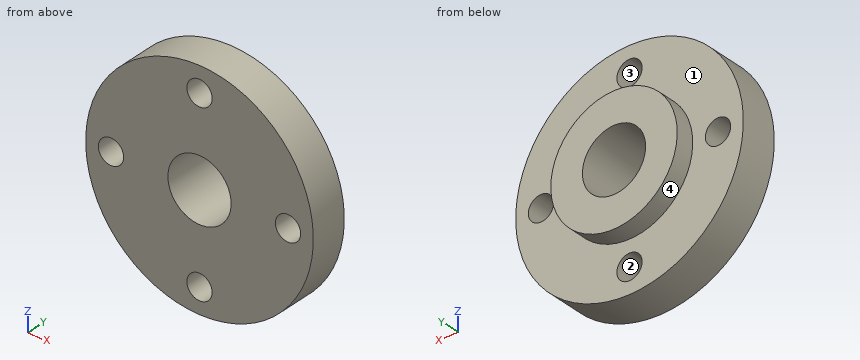
from build123d import *

# Parameters (mm, degrees)
SKETCH1_R           = 36
SKETCH1_R_2         = 10
BOSS_EXTRUDE1_DEPTH = 12
SKETCH2_R           = 20
SKETCH2_R_2         = 10
BOSS_EXTRUDE2_DEPTH = 6
CUT_EXTRUDE1_REACH  = 54.307
SKETCH3_R           = 4


with BuildPart() as part:
    # Sketch1 → Boss-Extrude1 (new body)
    with BuildSketch(Plane(origin=(0, 0, 0), x_dir=(1, 0, 0), z_dir=(0, 1, 0))):
        with Locations(Location((0, 0, 0), (0, 0, 270))):
            Circle(SKETCH1_R)
        with Locations(Location((0, 0, 0), (0, 0, 270))):
            Circle(SKETCH1_R_2, mode=Mode.SUBTRACT)
    extrude(amount=BOSS_EXTRUDE1_DEPTH)

    # Sketch2 → Boss-Extrude2 (add)
    with BuildSketch(Plane(origin=(0, 12, 0), x_dir=(1, 0, 0), z_dir=(0, 1, 0))):
        with Locations(Location((0, 0, 0), (0, 0, 270))):
            Circle(SKETCH2_R)
        with Locations(Location((0, 0, 0), (0, 0, 270))):
            Circle(SKETCH2_R_2, mode=Mode.SUBTRACT)
    extrude(amount=BOSS_EXTRUDE2_DEPTH)

    # Sketch3 → Cut-Extrude1 (cut, up to next)
    with BuildSketch(Plane(origin=(0, 12, 0), x_dir=(1, 0, 0), z_dir=(0, 1, 0)), mode=Mode.PRIVATE) as cut_extrude1_sk1:
        with Locations(Location((0, -28, 0), (0, 0, 270))):
            Circle(SKETCH3_R)
    cut_extrude1_tool1 = extrude(cut_extrude1_sk1.sketch, amount=-CUT_EXTRUDE1_REACH, mode=Mode.PRIVATE) & part.part
    # Sketch3 → Cut-Extrude1 (cut, up to next)
    with BuildSketch(Plane(origin=(0, 12, 0), x_dir=(1, 0, 0), z_dir=(0, 1, 0)), mode=Mode.PRIVATE) as cut_extrude1_sk2:
        with Locations(Location((-28, 0, 0), (0, 0, 270))):
            Circle(SKETCH3_R)
    cut_extrude1_tool2 = extrude(cut_extrude1_sk2.sketch, amount=-CUT_EXTRUDE1_REACH, mode=Mode.PRIVATE) & part.part
    # Sketch3 → Cut-Extrude1 (cut, up to next)
    with BuildSketch(Plane(origin=(0, 12, 0), x_dir=(1, 0, 0), z_dir=(0, 1, 0)), mode=Mode.PRIVATE) as cut_extrude1_sk3:
        with Locations(Location((0, 28, 0), (0, 0, 270))):
            Circle(SKETCH3_R)
    cut_extrude1_tool3 = extrude(cut_extrude1_sk3.sketch, amount=-CUT_EXTRUDE1_REACH, mode=Mode.PRIVATE) & part.part
    # Sketch3 → Cut-Extrude1 (cut, up to next)
    with BuildSketch(Plane(origin=(0, 12, 0), x_dir=(1, 0, 0), z_dir=(0, 1, 0)), mode=Mode.PRIVATE) as cut_extrude1_sk4:
        with Locations(Location((28, 0, 0), (0, 0, 270))):
            Circle(SKETCH3_R)
    cut_extrude1_tool4 = extrude(cut_extrude1_sk4.sketch, amount=-CUT_EXTRUDE1_REACH, mode=Mode.PRIVATE) & part.part
    add(cut_extrude1_tool1.solids().sort_by_distance((0, 12, 28))[0], mode=Mode.SUBTRACT)
    add(cut_extrude1_tool2.solids().sort_by_distance((-28, 12, 0))[0], mode=Mode.SUBTRACT)
    add(cut_extrude1_tool3.solids().sort_by_distance((0, 12, -28))[0], mode=Mode.SUBTRACT)
    add(cut_extrude1_tool4.solids().sort_by_distance((28, 12, 0))[0], mode=Mode.SUBTRACT)


solid = part.part
The listing builds one solid part. Answer for the finished solid, in the listing's coordinates (mm). Face numbers are marked on the shaded views. Give positions to 0.01 mm unless a question says otherwise; leave off trailing zeros. Order: outer loops, then holes, each group sorted by start corner. A loop starts at its lowest first (then second) coordinate and runs counter-clockwise, first axis right, second up. Notation, with made-up numbers: (23.5, -32.5) - (30.5, -32.5) arc R12 cw to (30.5, -11.5) - close; hole circle Ø7 at (-39, -16). An arc over 180 degrees is marked (long way). One line per item, written item: value. Start each with the question number.
1) A cutting plane is placed at D-D on x = -30.5. Give the vertices of the cut face in (y, z).
2) A cutting plane is placed at C-C on z = -28. Give the vertices of the cut face in (x, y), then the cut area to 3 significant figures.
3) Find the intervals of material crossed by L1, parallel to X at y = 8.75, z = 0; L2, parallel to X at y = 14, z = 0; L3, parallel to Z at x = -8, y = 4.5, in increasing order.
4) A cutting plane is placed at B-B on x = 0. Give the vertices of the cut face in (y, z), then the cut area to 3 significant figures.
5) A cutting plane is placed at A-A on z = 0. Give the vertices of the cut face in (x, y), then the cut area to 3 significant figures.
6) Given pin 1 Ø10.5 at (x, z) = (0, 28) entering from +Y; pin 2 Ø5 at (x, y) = (-9, 10) entering from +Z; pin 3 Ø8 at (y, z) = (9.5, 4) entering from -X; pin 4 Ø7 at (x, z) = (0, -28) entering from +Y, each flat-ended and moving along its own axis, determine where each tip first touches the part or whether it passes through.
7) The mould has two halves that part along Z. Classify the marked faces 1, 2, 3 and 4: released by +Z, released by -Z, zero draft, split by the parting line, or undercut.
Answer sheet:
1. outline: (0, -19.12) - (12, -19.12) - (12, -3.12) - (0, -3.12) - close; (0, 3.12) - (12, 3.12) - (12, 19.12) - (0, 19.12) - close
2. outline: (-22.63, 0) - (-4, 0) - (-4, 12) - (-22.63, 12) - close; (4, 0) - (22.63, 0) - (22.63, 12) - (4, 12) - close
2. area: 447 mm2
3. L1: x = -36 to -32, -24 to -10, 10 to 24, 32 to 36
3. L2: x = -20 to -10, 10 to 20
3. L3: z = -35.1 to -6, 6 to 35.1
4. outline: (0, -36) - (12, -36) - (12, -32) - (0, -32) - close; (0, -24) - (12, -24) - (12, -20) - (18, -20) - (18, -10) - (0, -10) - close; (0, 10) - (18, 10) - (18, 20) - (12, 20) - (12, 24) - (0, 24) - close; (0, 32) - (12, 32) - (12, 36) - (0, 36) - close
4. area: 552 mm2
5. outline: (-36, 0) - (-32, 0) - (-32, 12) - (-36, 12) - close; (-24, 0) - (-10, 0) - (-10, 18) - (-20, 18) - (-20, 12) - (-24, 12) - close; (10, 0) - (24, 0) - (24, 12) - (20, 12) - (20, 18) - (10, 18) - close; (32, 0) - (36, 0) - (36, 12) - (32, 12) - close
5. area: 552 mm2
6. pin 1: stops at y = 12
6. pin 2: stops at z = 35.41
6. pin 3: stops at x = -36
6. pin 4: passes through
7. face 1: zero draft
7. face 2: undercut
7. face 3: undercut
7. face 4: split by the parting line
